Design review of the part built by this model. Coordinates are the model's own, in mm. Round coordinates to 2 decimals unless told otherwise and drop trailing zeros. Write each loop counter-clockwise with the first axis right and the second up, starting at its lowest first coordinate (ties: lowest second). Pieces come first, ordered by that corner, then holes. Notation, with made-up numbers: (-25, 54.25) -> (7, 54.25) arc R9 ccw to (7, 61.25) -> close; hole circle Ø2 at (-27, 16). An arc over 180 degrees is marked (long way). One line per question, with ' | ' between items. Start each with the question number.
1) For probe 1 along Y at (x, z) = (0, 3.6); probe 2 along X at (y, z) = (-81.5, 1.8); probe 3 along Y at (x, z) = (-116.5, 1.65), list the stretches that pass through material, from the lowest coordinate up.
2) Insertion check: pin 1 Ø0.9 at (x, y) = (0, -7.2) entering from -Z; pin 2 Ø2.5 at (y, z) = (-90.5, 1.5) entering from +X; pin 3 Ø3 at (x, z) = (-85, 1.5) entering from +Y; pin 4 Ø2 at (y, z) = (-82.5, 3.5) entering from -X. Each pin has a flat end and moves straight along its axis. Give the tip position at first contact, or say it passes through.
3) Consider section B-B (z = 2). Count the separate pieces of the cut face and the enclosed holes in it, then the cut area to 3 significant figures.
4) Consider section A-A (y = -36). Give the boundary of the cut face in (x, z), then the cut area to 3 significant figures.
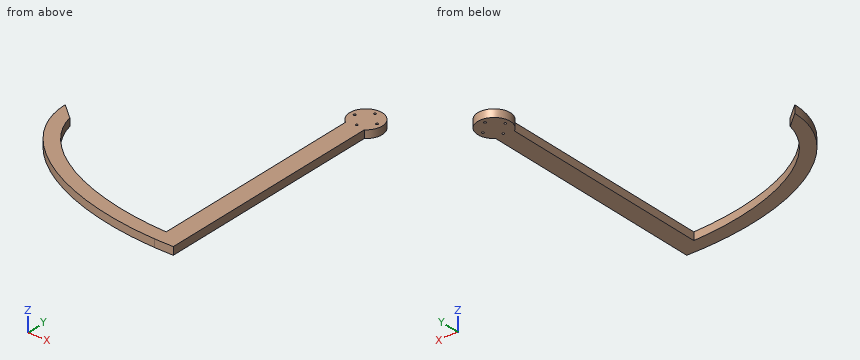
```python
from build123d import *

# Parameters (mm, degrees)
F0_R     = 10.5
F0_R_2   = 0.75
F1_DEPTH = 5
F3_DEPTH = 5


# Not quite as in the source:
# - a feature names something its author has since deleted; it is built from what else it names


with BuildPart() as f1:
    # F0 (on Top) → F1 (new body)
    with BuildSketch(Plane.XY):
        Circle(F0_R)
        with Locations((-3.45, -7.2)):
            Circle(F0_R_2, mode=Mode.SUBTRACT)
        with Locations((-7.2, -3.45)):
            Circle(F0_R_2, mode=Mode.SUBTRACT)
        with Locations((0, -7.2)):
            Circle(F0_R_2, mode=Mode.SUBTRACT)
        with Locations((3.45, -7.2)):
            Circle(F0_R_2, mode=Mode.SUBTRACT)
        with Locations((7.2, -3.45)):
            Circle(F0_R_2, mode=Mode.SUBTRACT)
        with Locations((-7.2, 0)):
            Circle(F0_R_2, mode=Mode.SUBTRACT)
        with Locations((-7.2, 3.45)):
            Circle(F0_R_2, mode=Mode.SUBTRACT)
        with Locations((-3.45, 7.2)):
            Circle(F0_R_2, mode=Mode.SUBTRACT)
        with Locations((7.2, 0)):
            Circle(F0_R_2, mode=Mode.SUBTRACT)
        with Locations((7.2, 3.45)):
            Circle(F0_R_2, mode=Mode.SUBTRACT)
        with Locations((0, 7.2)):
            Circle(F0_R_2, mode=Mode.SUBTRACT)
        with Locations((3.45, 7.2)):
            Circle(F0_R_2, mode=Mode.SUBTRACT)
        with Locations((3.45, -7.2)):
            Circle(F0_R_2)
        with Locations((-3.45, -7.2)):
            Circle(F0_R_2)
        with Locations((-7.2, -3.45)):
            Circle(F0_R_2)
        with Locations((-7.2, 3.45)):
            Circle(F0_R_2)
        with Locations((-3.45, 7.2)):
            Circle(F0_R_2)
        with Locations((3.45, 7.2)):
            Circle(F0_R_2)
        with Locations((7.2, 3.45)):
            Circle(F0_R_2)
        with Locations((7.2, -3.45)):
            Circle(F0_R_2)
    extrude(amount=F1_DEPTH)

    # F2 (on Top) → F3 (join, through all)
    with BuildSketch(Plane.XY):
        with BuildLine():
            Line((6, -8.7032937936), (6, -8.6168439698))
            Line((6, -8.6168439698), (-5.159e-07, -8.6168439698))
            add(Edge.make_bspline(
                [(6, -8.7032937936), (3.0017297357, -8.6168439624), (-5.159e-07, -8.6168439698)],
                knots=[4.6643705292, 4.6643705292, 4.6643705292, 4.7123889845, 4.7123889845, 4.7123889845], degree=2, weights=[1, 0.9997117923, 1]))
        make_face()
        with BuildLine():
            add(Edge.make_bspline(
                [(-5.159e-07, -8.6168439698), (-3.0017302513, -8.6168439772), (-6, -8.7032937936)],
                knots=[4.7123889845, 4.7123889845, 4.7123889845, 4.7604074315, 4.7604074315, 4.7604074315], degree=2, weights=[1, 0.9997117924, 1]))
            Line((-5.159e-07, -8.6168439698), (-6, -8.6168439698))
            Line((-6, -8.6168439698), (-6, -8.7032937936))
        make_face()
        with BuildLine():
            Line((6, -158.6168439698), (6, -158.530394146))
            add(Edge.make_bspline(
                [(0, -158.6168439698), (3.0017299935, -158.6168439698), (6, -158.530394146)],
                knots=[1.5707963268, 1.5707963268, 1.5707963268, 1.6188147779, 1.6188147779, 1.6188147779], degree=2, weights=[1, 0.9997117924, 1]))
            Line((0, -158.6168439698), (6, -158.6168439698))
        make_face()
        with BuildLine():
            Line((-6, -158.6168439698), (0, -158.6168439698))
            add(Edge.make_bspline(
                [(-6, -158.530394146), (-3.0017299935, -158.6168439698), (0, -158.6168439698)],
                knots=[1.5227778757, 1.5227778757, 1.5227778757, 1.5707963268, 1.5707963268, 1.5707963268], degree=2, weights=[1, 0.9997117924, 1]))
            Line((-6, -158.530394146), (-6, -158.6168439698))
        make_face()
        with BuildLine():
            add(Edge.make_bspline(
                [(0, -158.6168439698), (3.0017299935, -158.6168439698), (6, -158.530394146)],
                knots=[1.5707963268, 1.5707963268, 1.5707963268, 1.6188147779, 1.6188147779, 1.6188147779], degree=2, weights=[1, 0.9997117924, 1]))
            Line((6, -158.530394146), (6, -149.528497087))
            add(Edge.make_bspline(
                [(-6, -149.528497087), (0, -149.7053092713), (6, -149.528497087)],
                knots=[1.5190490974, 1.5190490974, 1.5190490974, 1.6225435562, 1.6225435562, 1.6225435562], degree=2, weights=[1, 0.9986614109, 1]))
            Line((-6, -149.528497087), (-6, -158.530394146))
            add(Edge.make_bspline(
                [(-6, -158.530394146), (-3.0017299935, -158.6168439698), (0, -158.6168439698)],
                knots=[1.5227778757, 1.5227778757, 1.5227778757, 1.5707963268, 1.5707963268, 1.5707963268], degree=2, weights=[1, 0.9997117924, 1]))
        make_face()
        with BuildLine():
            add(Edge.make_bspline(
                [(6, -8.7032937936), (3.0017297357, -8.6168439624), (-5.159e-07, -8.6168439698)],
                knots=[4.6643705292, 4.6643705292, 4.6643705292, 4.7123889845, 4.7123889845, 4.7123889845], degree=2, weights=[1, 0.9997117923, 1]))
            add(Edge.make_bspline(
                [(-5.159e-07, -8.6168439698), (-3.0017302513, -8.6168439772), (-6, -8.7032937936)],
                knots=[4.7123889845, 4.7123889845, 4.7123889845, 4.7604074315, 4.7604074315, 4.7604074315], degree=2, weights=[1, 0.9997117924, 1]))
            Line((-6, -8.7032937936), (-6, -17.7051908526))
            add(Edge.make_bspline(
                [(6, -17.7051908526), (0, -17.5283786684), (-6, -17.7051908526)],
                knots=[4.660641751, 4.660641751, 4.660641751, 4.7641362098, 4.7641362098, 4.7641362098], degree=2, weights=[1, 0.9986614109, 1]))
            Line((6, -17.7051908526), (6, -8.7032937936))
        make_face()
        with BuildLine():
            Line((6, -149.528497087), (6, -17.7051908526))
            add(Edge.make_bspline(
                [(6, -17.7051908526), (0, -17.5283786684), (-6, -17.7051908526)],
                knots=[4.660641751, 4.660641751, 4.660641751, 4.7641362098, 4.7641362098, 4.7641362098], degree=2, weights=[1, 0.9986614109, 1]))
            Line((-6, -17.7051908526), (-6, -149.528497087))
            add(Edge.make_bspline(
                [(-6, -149.528497087), (0, -149.7053092713), (6, -149.528497087)],
                knots=[1.5190490974, 1.5190490974, 1.5190490974, 1.6225435562, 1.6225435562, 1.6225435562], degree=2, weights=[1, 0.9986614109, 1]))
        make_face()
        with BuildLine():
            Line((-115.0107222667, -92.2180852847), (-125, -83.6168439698))
            add(Edge.make_bspline(
                [(-125, -83.6168439698), (-125, -155.0992391761), (-6, -158.530394146)],
                knots=[0, 0, 0, 1.5227778757, 1.5227778757, 1.5227778757], degree=2, weights=[1, 0.7238784428, 1]))
            Line((-6, -158.530394146), (-6, -149.528497087))
            add(Edge.make_bspline(
                [(-115.0107222667, -92.2180852847), (-102.427295797, -146.686910289), (-6, -149.528497087)],
                knots=[0.1306935792, 0.1306935792, 0.1306935792, 1.5190490974, 1.5190490974, 1.5190490974], degree=2, weights=[1, 0.7685799932, 1]))
        make_face()
    extrude(amount=F3_DEPTH)


solid = f1.part
```
From the geometry:
1) probe 1: y = -158.62 to -7.95, -6.45 to 6.45, 7.95 to 10.5 | probe 2: x = -6 to 6 | probe 3: y = -110.8 to -90.94
2) pin 1: passes through | pin 2: stops at x = 6 | pin 3: stops at y = -127.59 | pin 4: stops at x = -6
3) separate pieces: 1 | enclosed holes: 4 | area: 3,380 mm2
4) outline: (-6, 0) -> (6, 0) -> (6, 5) -> (-6, 5) -> close | area: 60.0 mm2
